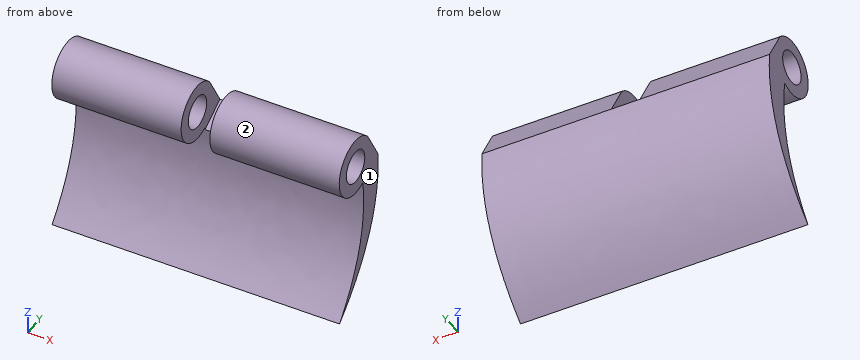
from build123d import *

# Parameters (mm, degrees)
SKETCH1_R           = 0.9
BOSS_EXTRUDE1_DEPTH = 16
SKETCH2_W           = 1.6
SKETCH2_H           = 4.200659695
CUT_EXTRUDE1_DEPTH  = 10


with BuildPart() as part:
    # Sketch1 → Boss-Extrude1 (new body)
    with BuildSketch(Plane(origin=(0, 0, 0), x_dir=(0, 0, -1), z_dir=(1, 0, 0))):
        with BuildLine():
            Line((-1.084501086, 1.173366689), (0.669981536, 2.201916273))
            add(Edge.make_bspline(
                [(0.669981536, 2.201916273), (5.142012003, 2.441554719), (8.521732168, -1.570541081)],
                knots=[0, 0, 0, 1, 1, 1], degree=2))
            add(Edge.make_bspline(
                [(1.429892444, 0.712979376), (5.328809075, 1.211697848), (8.521732168, -1.570541081)],
                knots=[0, 0, 0, 1, 1, 1], degree=2))
            ThreePointArc((1.429892444, 0.712979376), (-0.287772336, -1.571661247), (-1.084501086, 1.173366689))
        make_face()
        Circle(SKETCH1_R, mode=Mode.SUBTRACT)
    extrude(amount=BOSS_EXTRUDE1_DEPTH)

    # Sketch2 → Cut-Extrude1 (cut)
    with BuildSketch(Plane(origin=(0, 1.346412624, 0.789322234), x_dir=(1, 0, 0), z_dir=(0, 0.8626851476678137, 0.5057413726336444))):
        with Locations((8, -0.408746569)):
            Rectangle(SKETCH2_W, SKETCH2_H)
    extrude(amount=-CUT_EXTRUDE1_DEPTH, mode=Mode.SUBTRACT)


solid = part.part
Build history of the part. All positions in model axes, mm. Face numbers are marked on the shaded views. Round coordinates to 2 decimals unless told otherwise and drop trailing zeros. Order: outer loops, then holes, each group sorted by start corner. A loop starts at its lowest first (then second) coordinate and runs counter-clockwise, first axis right, second up. Notation, with made-up numbers: M 30,7.25 L 62,7.25 A11 cw 62,25.25 Z; hole C -14,27 d6. An arc over 180 degrees is marked long. Use CSV: the item, a comma, the result in double quotes. Start each with the question number.
(1) Cut at A-A on z = 0. List the corners of the cut face in (x, y).
(2) Flat gauge pins, fed straight in: P1, Ø1, axis at x = 10.5, z = -7, coming from the +Y side; P2, Ø1.5, axis at x = 10.5, z = -5, coming from the -Y side; P3, Ø3, axis at x = 4, z = -3.5, coming from the -Y side. Where does each tip first touch, or does it go through?
(3) Cut at B-B on y = 0.4. State how many separate pieces and enclosed holes the cut face has, then the cut area to 3 significant figures.
(4) Drill centre lines: probe 1 along Z at (x, y) = (7, -0.3); probe 2 along Z at (x, y) = (3, -0.2); probe 3 along X at (y, z) = (0.3, 1). Where is each one in solid material? Low to high.
(5) Mould opens along Z. For the marked faces 1 and 2 say: +Z half, -Z half, draft (parallel to the pull), parting line (faces both ways), or undercut.
Findings:
1,outline,"M 0,-1.6 L 7.2,-1.6 L 7.2,-0.9 L 0,-0.9 Z; M 0,0.9 L 7.2,0.9 L 7.2,1.81 L 0,1.81 Z; M 8.8,-1.6 L 16,-1.6 L 16,-0.9 L 8.8,-0.9 Z; M 8.8,0.9 L 16,0.9 L 16,1.81 L 8.8,1.81 Z"
2,P1,"stops at y = 0.38"
2,P2,"stops at y = 0.17"
2,P3,"stops at y = 0.44"
3,separate pieces,"5"
3,enclosed holes,"0"
3,area,"42.8 mm^2"
4,probe 1,"z = -7.31 to -6.73, -1.57 to -0.85, 0.85 to 1.57"
4,probe 2,"z = -7.2 to -6.55, -1.59 to -0.88, 0.88 to 1.59"
4,probe 3,"x = 0 to 7.2, 8.8 to 16"
5,face 1,"draft"
5,face 2,"undercut"
